Here's the drawing with two shaded views (mm, measured from the low corner). I have some questions. A direction names the side the tool comes from. Coordinates: 2 decimals unless noted, no trailing zeros. Loops run counter-clockwise (first coordinate to the right, second up) from the corner with the lowest first, then second, coordinate; pieces in that order, holes last. Notation, with made-up numbers: (86.25, 34) -> (109.25, 34) arc R26 cw to (109.25, 67) -> close; hole circle Ø2 at (21.5, 32.5). An arc over 180 degrees is marked (long way). Answer as a JSON object with one key per item and string values. Group by question number.
1) I'm going to push flat-ended pins straight in: pin 1 (12 mm diameter, centred on x = 20.5, y = 10, fed in from +Z); pin 2 (12 mm diameter, centred on x = 38, y = 8, fed in from +Z); pin 3 (2 mm diameter, centred on x = 32.5, z = 20.5, fed in from -Y); pin 4 (2 mm diameter, centred on x = 53, y = 11.5, fed in from +Z). Where does each tip first touch, or does it pass through?
2) I want a section at D-D (y = 14.5). Write out the boundary of the cut face in (x, z).
3) Which directions (+Z, -Z, +X, -X, +Y, -Y) give clear straight access to the entire face, cutting with the end or side of a thin tool? Please do the marked faces 4 and 5.
4) I want a section at B-B (y = 8). Write out the boundary of the cut face in (x, z).
5) I need wall thicknesses on probe 1 along X at (y, z) = (8, 20.5); probe 2 along Y at (x, z) = (22, 9.5); probe 3 along X at (y, z) = (4.5, 13.5). Which ranges of each line are inside material? Lowest first, please. Write a range as [from, to].
6) I want a section at A-A (z = 8.5). Write out the boundary of the cut face in (x, y).
7) If we mould it in two halves opening along X, with no side actions, what happens to the marked faces 1, 2 and 3? For each: +X half, -X half, draft (parallel to the pull), parting line (faces both ways), or undercut.
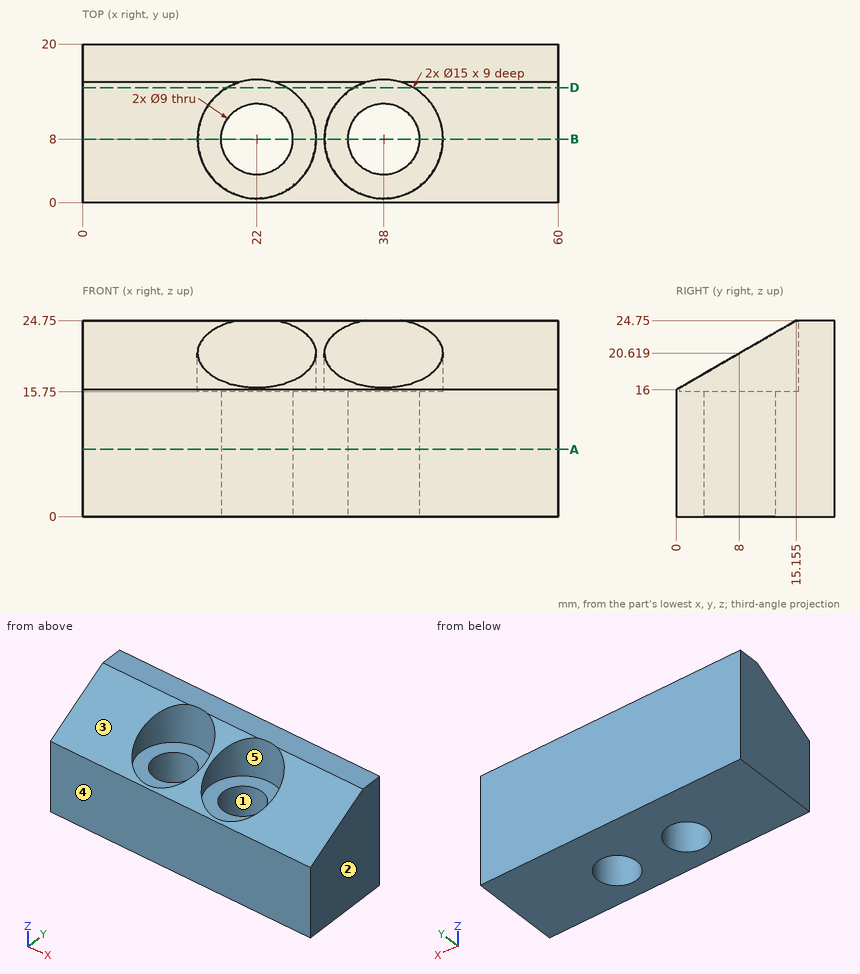
Determined:
{
 "1": {"pin 1": "z = 24.75", "pin 2": "z = 15.75", "pin 3": "y = 11.74", "pin 4": "z = 23.22"},
 "2": {"outline": "(0, 0) -> (60, 0) -> (60, 24.37) -> (41.74, 24.37) -> (41.74, 15.75) -> (34.26, 15.75) -> (34.26, 24.37) -> (25.74, 24.37) -> (25.74, 15.75) -> (18.26, 15.75) -> (18.26, 24.37) -> (0, 24.37) -> close"},
 "3": {"face 4": "+Z, -Z, +X, -X, -Y", "face 5": "+Z"},
 "4": {"outline": "(0, 0) -> (17.5, 0) -> (17.5, 15.75) -> (14.5, 15.75) -> (14.5, 20.62) -> (0, 20.62) -> close; (26.5, 0) -> (33.5, 0) -> (33.5, 15.75) -> (30.5, 15.75) -> (30.5, 20.62) -> (29.5, 20.62) -> (29.5, 15.75) -> (26.5, 15.75) -> close; (42.5, 0) -> (60, 0) -> (60, 20.62) -> (45.5, 20.62) -> (45.5, 15.75) -> (42.5, 15.75) -> close"},
 "5": {"probe 1": "[0, 14.5], [29.5, 30.5], [45.5, 60]", "probe 2": "[0, 3.5], [12.5, 20]", "probe 3": "[0, 19.17], [24.83, 35.17], [40.83, 60]"},
 "6": {"outline": "(0, 0) -> (60, 0) -> (60, 20) -> (0, 20) -> close; hole circle Ø9 at (22, 8); hole circle Ø9 at (38, 8)"},
 "7": {"face 1": "undercut", "face 2": "+X half", "face 3": "draft"}
}
